Could you check a few things on this model? Use its own coordinates, in mm. Face numbers are marked on the shaded views. A direction names the side the tool comes from. Coordinates: 2 decimals unless noted, no trailing zeros. Loops run counter-clockwise (first coordinate to the right, second up) from the corner with the lowest first, then second, coordinate; pieces in that order, holes last.
from build123d import *

# Parameters (mm, degrees)
EXTRUDE_2_DEPTH      = 20
EXTRUDE_2_2_DEPTH    = 60
CUT_EXTRUDE_2_DEPTH  = 52
FILLET_1_R           = 20
FILLET_2_R           = 10
FILLET_4_R           = 16
FILLET_5_R           = 16
M8X1_0_1_D           = 7
M8X1_0_1_CSINK_D     = 8.05
M8X1_0_1_CSINK_ANGLE = 90


with BuildPart() as part:
    # 草图1 → Extrude 2 (new body)
    with BuildSketch(Plane(origin=(0, 0, 0), x_dir=(1, 0, 0), z_dir=(0, 1, 0))):
        with BuildLine():
            Line((70, 71.414284285), (70, -71.414284285))
            ThreePointArc((70, -71.414284285), (-100, 0), (70, 71.414284285))
        make_face()
    extrude(amount=EXTRUDE_2_DEPTH)

    # 草图5 → Extrude 2 2 (add, symmetric)
    with BuildSketch(Plane.XY):
        Polygon((-55, 20), (-5, 106.602540378), (5.392304845, 100.602540378), (-44.607695155, 14), align=None)
    extrude(amount=EXTRUDE_2_2_DEPTH, both=True)

    # 草图7 → 切除-拉伸2 (cut, symmetric)
    with BuildSketch(Plane.XY):
        Polygon((-17.5, 84.951905284), (-7.107695155, 78.951905284), (-41.143593539, 20), (-55, 20), align=None)
    extrude(amount=CUT_EXTRUDE_2_DEPTH, both=True, mode=Mode.SUBTRACT)

    # 圆角1
    fillet_1_edges = [part.edges().sort_by_distance(p)[0] for p in [
        (0.196152423, 103.602540378, 60),
        (0.196152423, 103.602540378, -60),
    ]]
    fillet(fillet_1_edges, radius=FILLET_1_R)

    # 圆角2
    fillet_2_edges = [part.edges().sort_by_distance(p)[0] for p in [
        (-12.303847577, 81.951905284, -52),
        (-12.303847577, 81.951905284, 52),
    ]]
    fillet(fillet_2_edges, radius=FILLET_2_R)

    # 圆角4
    fillet_4_edges = [part.edges().sort_by_distance(p)[0] for p in [
        (-41.143593539, 20, -56),
    ]]
    fillet(fillet_4_edges, radius=FILLET_4_R)

    # 圆角5
    fillet_5_edges = [part.edges().sort_by_distance(p)[0] for p in [
        (-41.143593539, 20, 56),
    ]]
    fillet(fillet_5_edges, radius=FILLET_5_R)

    # M8x1.0 螺纹孔1 (through all)
    with Locations(Plane(origin=(0, 20, 0), x_dir=(1, 0, 0), z_dir=(0, 1, 0))):
        with Locations((-66.737936963, 0), (0, 66.737936963), (0, -66.737936963)):
            CounterSinkHole(M8X1_0_1_D / 2, M8X1_0_1_CSINK_D / 2, counter_sink_angle=M8X1_0_1_CSINK_ANGLE)


solid = part.part
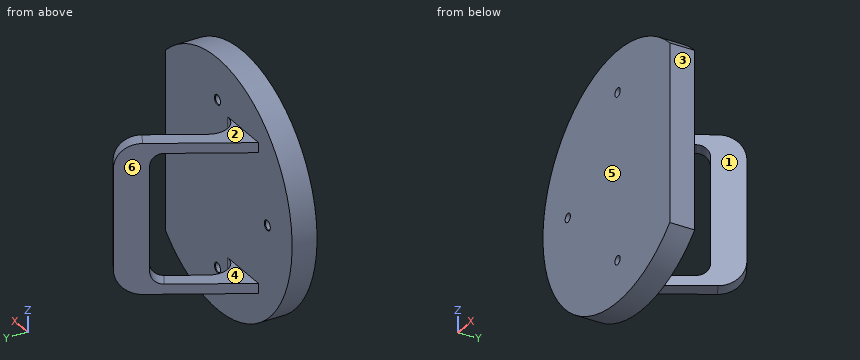
(1) Imagine slicing it at C-C, the plane y = 62. Write out the boundary of the cut face in (x, z), and give its area (3 significant figures).
Answers:
outline: (-30.75, -60) - (-16.89, -60) - (-16.89, -52) - (-30.75, -52) - close; (-30.75, 52) - (-16.89, 52) - (-16.89, 60) - (-30.75, 60) - close
area: 222 mm2
(2) I need wall thicknesses on probe 1 along Z at (x, y) = (0, 11.25); probe 2 along Y at (x, z) = (-32.5, -9.5); probe 3 along Z at (x, y) = (-6, 17). Which ranges of each line are inside material? Lowest first, please.
Answers:
probe 1: z = -100 to -70.24, -63.24 to 63.24, 70.24 to 100
probe 2: y = 0 to 20
probe 3: z = -99.82 to 99.82
(3) Imagine slicing it at A-A, the plane z = 0. Write out the boundary of the cut face in (x, y) (3 decimals), and give its area (3 significant figures).
Answers:
outline: (-100, 0) - (-70.238, 0) - (-70.238, 19.475) - (-70.763, 20) - (-100, 20) - close; (-63.238, 0) - (70, 0) - (70, 20) - (-62.713, 20) - (-63.238, 19.475) - close; (-17.5, 84.952) - (-7.108, 78.952) - (5.392, 100.603) - (-5, 106.603) - close
area: 3,560 mm2
(4) For pin 1 (13 mm diameter, centred on x = -30, y = 53.5, fed in from +Z); pin 2 (2 mm diameter, centred on x = -48, y = 23, fed in from -Z); pin 3 (12 mm diameter, centred on x = 7.5, z = -75.5, fed in from +Y); pin 4 (4 mm diameter, centred on x = -66.74, z = 0, fed in from +Y), each with a flat end and sliding along its axis, tell me the tip position at first contact or that it passes through.
Answers:
pin 1: stops at z = 60
pin 2: stops at z = -60
pin 3: stops at y = 20
pin 4: passes through
(5) Imagine slicing it at D-D, the plane x = 0. State how many separate pieces and enclosed holes the cut face has, and give its area (3 significant figures).
Answers:
separate pieces: 4
enclosed holes: 0
area: 5,030 mm2
(6) We'd pull the mould along Y, two halves only. Please class the marked faces 4, 5 and 6: +Y half, -Y half, draft (parallel to the pull), parting line (faces both ways), or undercut.
Answers:
face 4: undercut
face 5: -Y half
face 6: +Y half
(7) Which directions (+Z, -Z, +X, -X, +Y, -Y) give clear straight access to the entire face, cutting with the end or side of a thin tool? Please do the marked faces 1, 2 and 3.
Answers:
face 1: +Z, -Z, +X
face 2: +Z, +X, -X, +Y
face 3: +Z, -Z, +X, +Y, -Y
(8) Imagine slicing it at B-B, the plane z = -27. Write out the boundary of the cut face in (x, y), and give its area (3 significant figures).
Answers:
outline: (-96.29, 0) - (70, 0) - (70, 20) - (-96.29, 20) - close; (-17.5, 84.95) - (-7.11, 78.95) - (5.39, 100.6) - (-5, 106.6) - close
area: 3,630 mm2
